Geometry: see drawing. Coordinates: mm, zero at the bounding-box minimum. Give positions to 0.01 mm unless a question says otherwise; leave off trailing zeros. Write each loop counter-clockwise with the first axis right and the second up, starting at its lowest first coordinate (ties: lowest second). Pieces come first, ordered by that corner, then holes.
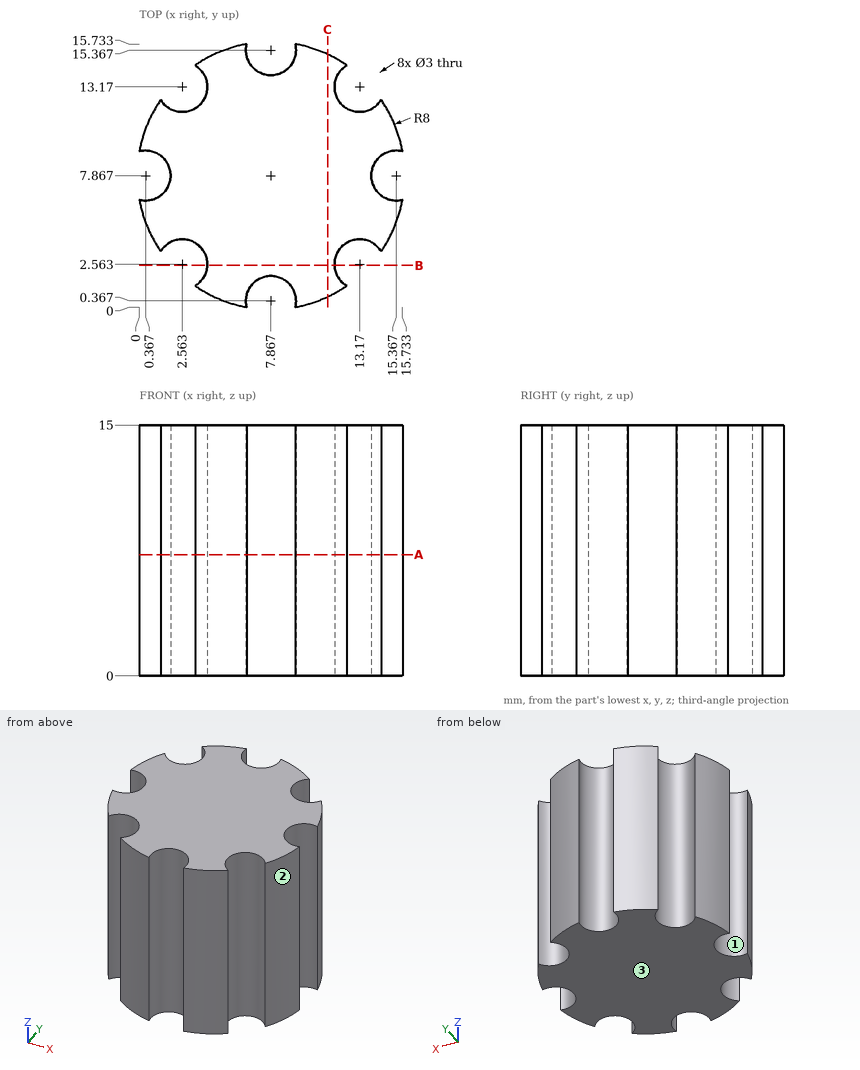
Q1. Section C-C, the plane x = 11.25. Return the cut outline in (y, z).
Q2. Pin query (flat end, axial travel): pin 1 (3.5 mm diameter, centred on x = 0.37, y = 7.87, fed in from -Z); pin 2 (2.5 mm diameter, centred on x = 2.56, y = 13.17, fed in from -Z); pin 3 (1.5 mm diameter, centred on y = 8, z = 10.5, fed in from +X) (1 decimal); pin 4 (3 mm diameter, centred on x = 11, z = 4, fed in from +Y). Return the tip coordinate at first contact, or that it passes through.
Q3. Section A-A, the plane z = 7.25. Return the cut outline in (x, y) (1 decimal), then the cut area to 3 significant figures.
Q4. Mould query, pull axis Y, two halves, no side actions, for the marked faces 1, 2 and 3. Classes: +Y half, -Y half, draft (parallel to the pull), parting line (faces both ways), or undercut.
Q5. Material intervals for line 1 along X through (y, z) = (3.5, 10.75) (1 decimal); line 2 along X through (y, z) = (2.5, 1.75); line 3 along X through (y, z) = (14.25, 10.75) (1 decimal), sorted ascending.
Q6. Section B-B, the plane y = 2.5. Return the cut outline in (x, z), then the cut area to 3 significant figures.
Solutions:
1. outline: (0.62, 0) - (15.12, 0) - (15.12, 15) - (0.62, 15) - close
2. pin 1: stops at z = 0
2. pin 2: passes through
2. pin 3: stops at x = 14.2
2. pin 4: stops at y = 15.7
3. outline: (0, 6.4) arc R8 ccw to (1.3, 3.3) arc R1.5 cw (long way) to (3.3, 1.3) arc R8 ccw to (6.4, 0) arc R1.5 cw (long way) to (9.3, 0) arc R8 ccw to (12.4, 1.3) arc R1.5 cw (long way) to (14.5, 3.3) arc R8 ccw to (15.7, 6.4) arc R1.5 cw (long way) to (15.7, 9.3) arc R8 ccw to (14.5, 12.4) arc R1.5 cw (long way) to (12.4, 14.5) arc R8 ccw to (9.3, 15.7) arc R1.5 cw (long way) to (6.4, 15.7) arc R8 ccw to (3.3, 14.5) arc R1.5 cw (long way) to (1.3, 12.4) arc R8 ccw to (0, 9.3) arc R1.5 cw (long way) to start
3. area: 162 mm2
4. face 1: undercut
4. face 2: -Y half
4. face 3: draft
5. line 1: x = 1.2 to 1.4, 3.7 to 12, 14.3 to 14.6
5. line 2: x = 4.06 to 11.67
5. line 3: x = 3.6 to 6.9, 8.9 to 12.1
6. outline: (4.06, 0) - (11.67, 0) - (11.67, 15) - (4.06, 15) - close
6. area: 114 mm2
